Design review of the part built by this model. Coordinates are the model's own, in mm. A direction names the side the tool comes from. Give positions to 0.01 mm unless a question says otherwise; leave off trailing zeros. Loops run counter-clockwise (first coordinate to the right, second up) from the corner with the lowest first, then second, coordinate; pieces in that order, holes last. Notation, with made-up numbers: M 48,61 L 103,61 A25 ccw 103,96 Z; hole C 81,-25.5 d1. An arc over 180 degrees is marked long. Use a Markdown table: item, result. Add a question column.
(1) Add section C-C, the plane z = 16.5. State how many separate pieces and enclosed holes the cut face has, then the cut area to 3 significant figures.
(2) Add section D-D, the plane y = -4. Give the boundary of the cut face in (x, z) (3 decimals), then the cut area to 3 significant figures.
(3) For faces 1 (the face through (22.2, -33.5, 30.1)), 2 (the face through (19.1, -20, 13.5)), 3 (the face through (10.267, -31.124, 35.249)), list the 3-axis set-ups (+Z, -Z, +X, -X, +Y, -Y) from which the entire face can be reached by the end or side of a thin tool; tool diameter is ignored.
(4) Add section A-A, the plane z = 33. Give the boundary of the cut face in (x, y).
(5) For probe 1 along Y at (x, z) = (6, 13); probe 2 along X at (y, z) = (-18, 21); probe 3 along Y at (x, z) = (8, 13.5), list the stretches that pass through material, from the lowest coordinate up.
(6) Insertion check: pin 1 Ø1.5 at (x, y) = (12.5, -18) entering from +Z (3 decimals); pin 2 Ø3 at (y, z) = (-9, 14) entering from +X; pin 3 Ø2 at (x, z) = (22, 10.5) entering from -Y. Each pin has a flat end and moves straight along its axis. Give the tip position at first contact, or say it passes through.
(7) Draft analysis for pull direction Y (two halves, no side actions). For faces 4 (the face through (9.49, -12.89, 13.74)), 5 (the face through (12.7, -15, 21)), 6 (the face through (24.7, -15.24, 18)), state which applies: pulls with the +Y half, pulls with the -Y half, needs draft (parallel to the pull), parting line crosses it, or undercut.
```python
from build123d import *

# Parameters (mm, degrees)
F0_W      = 38.1
F0_H      = 38.1
F1_DEPTH  = 38.1
F6_DEPTH  = 38.1
F8_DEPTH  = 38.1
F9_W      = 25.4
F9_H      = 7.62
F10_DEPTH = 38.1


with BuildPart() as f1:
    # F0 (on Front) → F1 (new body)
    with BuildSketch(Plane.XZ):
        with Locations((19.05, 19.05)):
            Rectangle(F0_W, F0_H)
    extrude(amount=F1_DEPTH)

    # F5 (on offset) → F6 (cut)
    with BuildSketch(Plane.YZ.offset(38.1)):
        Polygon((-11.43, 15.253705), (-7.626852, 38.1), (-31.75, 38.1), (-26.67, 14.965899), (-21.59, 28.575), (-16.51, 28.575), align=None)
        Polygon((-31.75, 0), (-38.1, 38.1), (-38.1, 0), align=None)
        Polygon((-25.4, 0), (-12.7, 0), (-19.05, 15.875), align=None)
        Polygon((-6.35, 0), (0, 0), (0, 38.1), align=None)
    extrude(amount=-F6_DEPTH, mode=Mode.SUBTRACT)

    # F7 (on offset) → F8 (cut)
    with BuildSketch(Plane.XZ.offset(38.1)):
        Polygon((6.35, 38.1), (0, 38.1), (0, 0), align=None)
        Polygon((25.4, 38.1), (12.7, 38.1), (19.05, 22.225), align=None)
        Polygon((38.1, 38.1), (31.75, 38.1), (38.1, 0), align=None)
        Polygon((11.43, 22.225), (6.35, 0), (31.75, 0), (26.67, 22.225), (21.59, 9.525), (16.51, 9.525), align=None)
    extrude(amount=-F8_DEPTH, mode=Mode.SUBTRACT)

    # F9 (on offset) → F10 (cut)
    with BuildSketch(Plane.XY.offset(38.1)):
        with Locations((25.4, -11.43)):
            Rectangle(F9_W, F9_H)
        with Locations((12.7, -26.67)):
            Rectangle(F9_W, F9_H)
    extrude(amount=-F10_DEPTH, mode=Mode.SUBTRACT)


solid = f1.part
```
Established:
| question | item | result |
|---|---|---|
| 1 | separate pieces | 9 |
| 1 | enclosed holes | 0 |
| 1 | area | 498 mm^2 |
| 2 | outline | M 2.35,14.1 L 9.573,14.1 L 11.43,22.225 L 14.68,14.1 L 23.42,14.1 L 26.67,22.225 L 28.527,14.1 L 35.75,14.1 L 31.75,38.1 L 25.4,38.1 L 19.05,22.225 L 12.7,38.1 L 6.35,38.1 Z |
| 2 | area | 563 mm^2 |
| 3 | face 1 | +Z, +Y, -Y |
| 3 | face 2 | -Z, +X, -X |
| 3 | face 3 | +Z, +X, -X |
| 4 | outline | M 5.5,-37.25 L 14.74,-37.25 L 14.74,-30.63 L 5.5,-30.63 Z; M 5.5,-8.48 L 12.7,-8.48 L 12.7,-7.62 L 14.74,-7.62 L 14.74,-0.85 L 5.5,-0.85 Z; M 23.36,-37.25 L 32.6,-37.25 L 32.6,-30.63 L 23.36,-30.63 Z; M 23.36,-7.62 L 32.6,-7.62 L 32.6,-0.85 L 23.36,-0.85 Z |
| 5 | probe 1 | -33.92 to -30.48, -22.86 to -20.2, -17.9 to -4.18 |
| 5 | probe 2 | 3.5 to 11.15, 11.92 to 26.18, 26.95 to 34.6 |
| 5 | probe 3 | -34 to -30.48, -22.86 to -20, -18.1 to -4.1 |
| 6 | pin 1 | z = 28.575 |
| 6 | pin 2 | x = 35.86 |
| 6 | pin 3 | y = -33.67 |
| 7 | face 4 | needs draft |
| 7 | face 5 | undercut |
| 7 | face 6 | undercut |
